Verification items for the finished model (mm, model axes). Face numbers are marked on the shaded views. A direction names the side the tool comes from. Give positions to 0.01 mm unless a question says otherwise; leave off trailing zeros. Write each loop counter-clockwise with the first axis right and the second up, starting at its lowest first coordinate (ties: lowest second). Pieces come first, ordered by that corner, then holes.
from build123d import *

# Parameters (mm, degrees)
ESQUISSE1_W             = 54
ESQUISSE1_H             = 46
MAIN_DEPTH              = 7.5
ESQUISSE2_R             = 1.35
USBFIXHOLES_DEPTH       = 8.5
ESQUISSE3_R             = 5
CIRCLESUPPORT_DEPTH     = 3
ESQUISSE4_W             = 45
ESQUISSE4_H             = 10.5
SIDECUTOFF_DEPTH        = 6
ESQUISSE6_W             = 45
ESQUISSE6_H             = 10.5
SIDELEFTCUTOFF_DEPTH    = 6
ESQUISSE7_W             = 2.9
ESQUISSE7_H             = 34
MAKERBEAMFIXSHAFT_DEPTH = 1
ESQUISSE10_W            = 42
ESQUISSE10_H            = 22
CENTRALHOLE_DEPTH       = 1
CENTRALHOLE_DEPTH_BACK  = 11.5
VERTICALFIXHOLE_REACH   = 57
ESQUISSE8_R             = 1.5
ESQUISSE11_R            = 1.35
USBFIXHOLES2_DEPTH      = 4


with BuildPart() as part:
    # Esquisse1 → Main (new body)
    with BuildSketch(Plane.XY):
        Rectangle(ESQUISSE1_W, ESQUISSE1_H)
    extrude(amount=MAIN_DEPTH)

    # Esquisse2 → UsbFixHoles (cut, through all)
    with BuildSketch(Plane.XY.offset(7.5)):
        with Locations((-22, -12)):
            Circle(ESQUISSE2_R)
        with Locations((-22, 12)):
            Circle(ESQUISSE2_R)
        with Locations((21.5, 18)):
            Circle(ESQUISSE2_R)
        with Locations((21.5, -18)):
            Circle(ESQUISSE2_R)
    extrude(amount=-USBFIXHOLES_DEPTH, mode=Mode.SUBTRACT)

    # Esquisse3 → CircleSupport (add)
    with BuildSketch(Plane.XY.offset(7.5)):
        with Locations((-22, 12)):
            Circle(ESQUISSE3_R)
        with Locations((-22, -12)):
            Circle(ESQUISSE3_R)
        with Locations((21.5, -18)):
            Circle(ESQUISSE3_R)
        with Locations((21.5, 18)):
            Circle(ESQUISSE3_R)
    extrude(amount=CIRCLESUPPORT_DEPTH)

    # Esquisse4 → SideCutoff (cut)
    with BuildSketch(Plane.XZ.offset(23)):
        with Locations((-4.5, 5.25)):
            Rectangle(ESQUISSE4_W, ESQUISSE4_H)
    extrude(amount=-SIDECUTOFF_DEPTH, mode=Mode.SUBTRACT)

    # Esquisse6 → SideLeftCutoff (cut)
    with BuildSketch(Plane(origin=(0, 23, 0), x_dir=(1, 0, 0), z_dir=(0, 1, 0))):
        with Locations((-4.5, -5.25)):
            Rectangle(ESQUISSE6_W, ESQUISSE6_H)
    extrude(amount=-SIDELEFTCUTOFF_DEPTH, mode=Mode.SUBTRACT)

    # Esquisse7 → MakerBeamFixShaft (add)
    with BuildSketch(Plane.ZY.offset(27)):
        with Locations((2.5, 0)):
            Rectangle(ESQUISSE7_W, ESQUISSE7_H)
    extrude(amount=MAKERBEAMFIXSHAFT_DEPTH)

    # Esquisse10 → CentralHole (cut, two sides)
    with BuildSketch(Plane.XY.offset(10.5)) as centralhole_sk:
        Rectangle(ESQUISSE10_W, ESQUISSE10_H)
    extrude(amount=CENTRALHOLE_DEPTH, mode=Mode.SUBTRACT)
    extrude(centralhole_sk.sketch, amount=-CENTRALHOLE_DEPTH_BACK, mode=Mode.SUBTRACT)

    # Esquisse8 → VerticalFixHole (cut, up to next)
    with BuildSketch(Plane.ZY.offset(28), mode=Mode.PRIVATE) as verticalfixhole_sk1:
        with Locations((2.5, 0)):
            Circle(ESQUISSE8_R)
    verticalfixhole_tool1 = extrude(verticalfixhole_sk1.sketch, amount=-VERTICALFIXHOLE_REACH, mode=Mode.PRIVATE) & part.part
    add(verticalfixhole_tool1.solids().sort_by_distance((-28, 0, 2.5))[0], mode=Mode.SUBTRACT)

    # Esquisse11 → UsbFixHoles2 (cut, through all)
    with BuildSketch(Plane(origin=(0, 0, 7.5), x_dir=(-1, 0, 0), z_dir=(0, 0, -1))):
        with Locations((-21.5, 18)):
            Circle(ESQUISSE11_R)
        with Locations((22, 12)):
            Circle(ESQUISSE11_R)
        with Locations((22, -12)):
            Circle(ESQUISSE11_R)
        with Locations((-21.5, -18)):
            Circle(ESQUISSE11_R)
    extrude(amount=-USBFIXHOLES2_DEPTH, mode=Mode.SUBTRACT)


solid = part.part
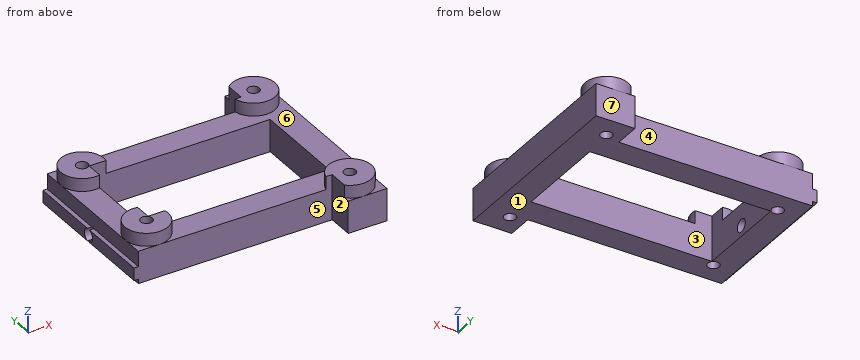
Item 1: Set-up check for the marked faces 1, 2, 3 and 4: record each of +Z, -Z, +X, -X, +Y, -Y from which the full face is reachable in a straight line by a thin tool's end or side.
Answer key:
face 1: -Z, +X, -X, +Y, -Y
face 2: +Z, -Z, -X, -Y
face 3: +Z, -Z
face 4: +Z, -Z, -X, +Y
Item 2: Depth check by flat-ended pin: pin 1 (4 mm diameter, centred on x = -16.5, z = 2, fed in from -Y); pin 2 (3 mm diameter, centred on x = -23, y = 1, fed in from +Z); pin 3 (0.5 mm diameter, centred on x = -27.5, y = 7, fed in from +Z). Enter the tip coordinate at first touch or a pass-through.
Answer key:
pin 1: stops at y = -17
pin 2: stops at z = 7.5
pin 3: stops at z = 3.95
Item 3: Sectioned sample at C-C on z = 2.5. Record the cut outline in (x, y), then the cut area to 3 significant figures.
Answer key:
outline: (-28, -17) - (18, -17) - (18, -23) - (27, -23) - (27, 23) - (18, 23) - (18, 17) - (-28, 17) - (-28, 1.5) - (-21, 1.5) - (-21, 11) - (21, 11) - (21, -11) - (-21, -11) - (-21, -1.5) - (-28, -1.5) - close; hole circle Ø2.7 at (-22, -12); hole circle Ø2.7 at (-22, 12); hole circle Ø2.7 at (21.5, -18); hole circle Ø2.7 at (21.5, 18)
area: 1,010 mm2
Item 4: Release check for a two-part mould opening along Y. For the marked faces 5, 6 and 7 record: released by +Y, released by -Y, zero draft, split by the parting line, or undercut.
Answer key:
face 5: released by -Y
face 6: undercut
face 7: released by +Y
Item 5: Scan lines: line 1 along Y through (x, z) = (-22, 8.3); line 2 along Y through (x, z) = (21.5, 4); line 3 along X through (y, z) = (0, 4.25). Record each from-to range of solid material in increasing order.
Answer key:
line 1: y = -17 to -13.35, -10.65 to -7, 7 to 10.65, 13.35 to 17
line 2: y = -23 to -19.35, -16.65 to 16.65, 19.35 to 23
line 3: x = -27 to -21, 21 to 27
Item 6: Sectioned sample at A-A on y = -5. Record the cut outline in (x, z).
Answer key:
outline: (-28, 1.05) - (-27, 1.05) - (-27, 0) - (-21, 0) - (-21, 7.5) - (-27, 7.5) - (-27, 3.95) - (-28, 3.95) - close; (21, 0) - (27, 0) - (27, 7.5) - (21, 7.5) - close
Item 7: Sectioned sample at B-B on x = -6. Record the cut outline in (y, z), then the cut area to 3 significant figures.
Answer key:
outline: (-17, 0) - (-11, 0) - (-11, 7.5) - (-17, 7.5) - close; (11, 0) - (17, 0) - (17, 7.5) - (11, 7.5) - close
area: 90.0 mm2
Item 8: Sectioned sample at D-D on y = -18. Record the cut outline in (x, z).
Answer key:
outline: (18, 0) - (20.15, 0) - (20.15, 10.5) - (18, 10.5) - close; (22.85, 0) - (27, 0) - (27, 7.5) - (26.5, 7.5) - (26.5, 10.5) - (22.85, 10.5) - close
